```python
from build123d import *

# Parameters (mm, degrees)
SKETCH_2_W          = 460
SKETCH_2_H          = 110
EXTRUDE_1_DEPTH     = 8
SKETCH_4_R          = 1.5
CUT_EXTRUDE_1_DEPTH = 237.619948441
SKETCH_3_R          = 2.5
SKETCH_3_R_2        = 1.5
CUT_EXTRUDE_2_DEPTH = 237.619948441
FILLET_1_R          = 10
SKETCH_5_W          = 60
SKETCH_5_H          = 20
SKETCH_5_W_2        = 40
CUT_EXTRUDE_3_DEPTH = 237.619948441


with BuildPart() as part:
    # 草图2 → 凸台-拉伸1 (new body)
    with BuildSketch(Plane(origin=(0, 0, 0), x_dir=(1, 0, 0), z_dir=(0, 1, 0))):
        Rectangle(SKETCH_2_W, SKETCH_2_H)
    extrude(amount=EXTRUDE_1_DEPTH)

    # 草图4 → 切除-拉伸1 (cut, through all)
    with BuildSketch(Plane(origin=(0, 8, 0), x_dir=(1, 0, 0), z_dir=(0, 1, 0))):
        with Locations(Location((-70, 35, 0), (0, 0, 270))):
            Circle(SKETCH_4_R)
        with Locations(Location((-70, -23, 0), (0, 0, 270))):
            Circle(SKETCH_4_R)
        with Locations(Location((-215, -23, 0), (0, 0, 270))):
            Circle(SKETCH_4_R)
        with Locations(Location((-215, 40, 0), (0, 0, 270))):
            Circle(SKETCH_4_R)
        with Locations(Location((-170, -23, 0), (0, 0, 270))):
            Circle(SKETCH_4_R)
        with Locations(Location((-215, 8.5, 0), (0, 0, 270))):
            Circle(SKETCH_4_R)
    cut_extrude_1 = extrude(amount=-CUT_EXTRUDE_1_DEPTH, mode=Mode.SUBTRACT)

    # 草图3 → 切除-拉伸2 (cut, through all)
    with BuildSketch(Plane(origin=(0, 8, 0), x_dir=(1, 0, 0), z_dir=(0, 1, 0))):
        with Locations(Location((-120, 35, 0), (0, 0, 270))):
            Circle(SKETCH_3_R)
        with Locations(Location((-120, 15, 0), (0, 0, 270))):
            Circle(SKETCH_3_R)
        with Locations(Location((-152, 32.5, 0), (0, 0, 270))):
            Circle(SKETCH_3_R_2)
        with Locations(Location((-152, 22.5, 0), (0, 0, 270))):
            Circle(SKETCH_3_R_2)
        with Locations(Location((-96, 32.5, 0), (0, 0, 270))):
            Circle(SKETCH_3_R_2)
        with Locations(Location((-96, 22.5, 0), (0, 0, 270))):
            Circle(SKETCH_3_R_2)
        with Locations(Location((-120, -10, 0), (0, 0, 270))):
            Circle(SKETCH_3_R)
        Polygon((-70, 55), (-48.5526258, 35), (48.5526258, 35), (70, 55), align=None)
    cut_extrude_2 = extrude(amount=-CUT_EXTRUDE_2_DEPTH, mode=Mode.SUBTRACT)

    # 镜向1: 切除-拉伸1, 切除-拉伸2 across plane
    add(cut_extrude_1.mirror(Plane(origin=(0, 0, 0), x_dir=(0, 0, 1), z_dir=(1, 0, 0))), mode=Mode.SUBTRACT)
    add(cut_extrude_2.mirror(Plane(origin=(0, 0, 0), x_dir=(0, 0, 1), z_dir=(1, 0, 0))), mode=Mode.SUBTRACT)

    # 圆角1
    fillet_1_edges = [part.edges().sort_by_distance(p)[0] for p in [
        (-70, 4, -55),
        (70, 4, -55),
        (48.5526258, 4, -35),
        (-48.5526258, 4, -35),
        (-230, 4, -55),
        (230, 4, -55),
    ]]
    fillet(fillet_1_edges, radius=FILLET_1_R)

    # 草图5 → 切除-拉伸3 (cut, through all)
    with BuildSketch(Plane(origin=(0, 8, 0), x_dir=(1, 0, 0), z_dir=(0, 1, 0))):
        with Locations((0, -45)):
            Rectangle(SKETCH_5_W, SKETCH_5_H)
        with Locations((120, -45)):
            Rectangle(SKETCH_5_W_2, SKETCH_5_H)
    cut_extrude_3 = extrude(amount=-CUT_EXTRUDE_3_DEPTH, mode=Mode.SUBTRACT)

    # 镜向2: 切除-拉伸3 across plane
    add(cut_extrude_3.mirror(Plane(origin=(0, 0, 0), x_dir=(0, 0, 1), z_dir=(1, 0, 0))), mode=Mode.SUBTRACT)


solid = part.part
```
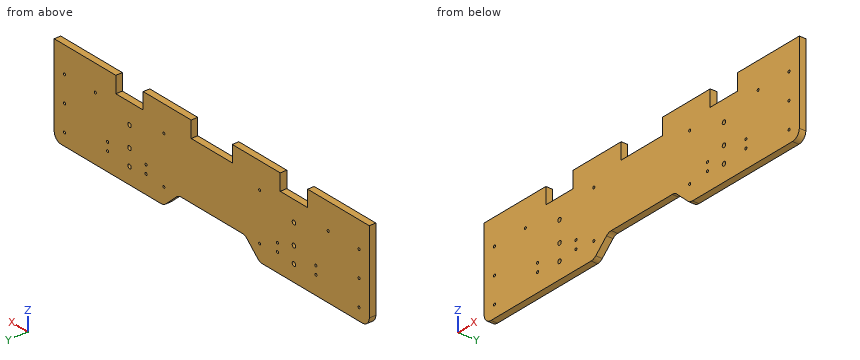
Input: part model. Units: mm. Frame: model coordinates. Give positions to 0.01 mm unless a question says otherwise; leave off trailing zeros. Order: outer loops, then holes, each group sorted by start corner. A loop starts at its lowest first (then second) coordinate and runs counter-clockwise, first axis right, second up. Notation, with made-up numbers: M -7,21.25 L 29,21.25 A19 cw 29,44.25 Z; hole C 86,-17.5 d3. An arc over 180 degrees is marked long. Return JSON: item names as keys, results as strings.
1) Section query A-A on y = 5.5. Count the separate pieces of the cut face and the enclosed holes in it, and give its area (3 significant figures).
Taken from the geometry:
{"separate pieces": "1", "enclosed holes": "26", "area": "45,100 mm2"}
2) Contact query for flat-ended pins moving along their axis: pin 1 (4 mm diameter, centred on x = -120.5, y = 2, fed in from +Z); pin 2 (3 mm diameter, centred on x = 120, z = -35, fed in from +Y); pin 3 (2 mm diameter, centred on x = 16, y = 2.5, fed in from -Z). Output: stop coordinate, or through.
Taken from the geometry:
{"pin 1": "stops at z = 35", "pin 2": "passes through", "pin 3": "stops at z = -35"}
3) Section query B-B on x = -10. Output: boundary loops of the cut face in (y, z).
Taken from the geometry:
{"outline": "M 0,-35 L 8,-35 L 8,35 L 0,35 Z"}
4) Line query: L1, parallel to X at y = 4.25, z = -15; L2, parallel to X at y = 2.5, z = -22; L3, parallel to X at y = 3, z = 36.5. Output: solid intervals per line, ascending. Write a range as [from, to].
Taken from the geometry:
{"L1": "x = [-230, -122.5], [-117.5, 117.5], [122.5, 230]", "L2": "x = [-230, -153.41], [-150.59, -97.41], [-94.59, 94.59], [97.41, 150.59], [153.41, 230]", "L3": "x = [-230, -140], [-100, -30], [30, 100], [140, 230]"}
